Input: part model. Units: mm. Frame: model coordinates. Face numbers are marked on the shaded views. Give positions to 0.01 mm unless a question says otherwise; leave off trailing zeros. Loops run counter-clockwise (first coordinate to the right, second up) from the corner with the lowest first, then second, coordinate; pieces in that order, holes last. Notation, with made-up numbers: (-10.75, -38) - (-6.75, -38) arc R22 ccw to (-6.75, -22) - close; hole circle Ø5 at (64, 57). An arc over 180 degrees is marked (long way). Answer as a JSON object with one key per item and string values.
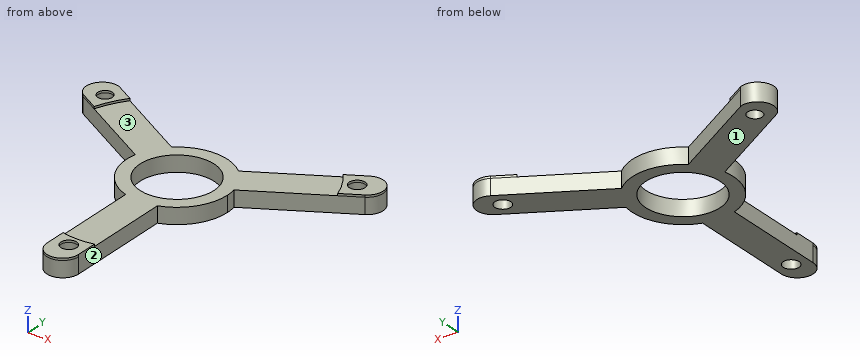
from build123d import *

# Parameters (mm, degrees)
F1_R     = 7.0078592828
F2_DEPTH = 3
F3_R     = 1.3785641614
F3_R_2   = 1.5
F4_DEPTH = 25
F5_R     = 1.3785641614
F5_R_2   = 1.5
F6_DEPTH = 0.4


# Not quite as in the source:
# - a feature names something its author has since deleted; it is built from what else it names


with BuildPart() as f2:
    # F1 (on Top) → F2 (new body)
    with BuildSketch(Plane.XY):
        with BuildLine():
            ThreePointArc((6.3250837122, 7.115890399), (8.2451158332, 4.7603198458), (9.3250837122, 1.9197379763))
            Line((9.3250837122, 1.9197379763), (26.6455917878, 11.9197379763))
            ThreePointArc((26.6455917878, 11.9197379763), (27.7436679992, 16.0178141876), (23.6455917878, 17.115890399))
            Line((23.6455917878, 17.115890399), (6.3250837122, 7.115890399))
        make_face()
        with BuildLine():
            Line((3, -29.0356283753), (3, -9.0356283753))
            ThreePointArc((3, -9.0356283753), (0, -9.5206396916), (-3, -9.0356283753))
            Line((-3, -9.0356283753), (-3, -29.0356283753))
            ThreePointArc((-3, -29.0356283753), (0, -32.0356283753), (3, -29.0356283753))
        make_face()
        with BuildLine():
            ThreePointArc((3, -9.0356283753), (7.7202493228, -5.5713849742), (9.5206396916, 0))
            ThreePointArc((9.5206396916, 0), (9.4716245242, 0.9648362606), (9.3250837122, 1.9197379763))
            ThreePointArc((9.3250837122, 1.9197379763), (8.2451158332, 4.7603198458), (6.3250837122, 7.115890399))
            ThreePointArc((6.3250837122, 7.115890399), (0, 9.5206396916), (-6.3250837122, 7.115890399))
            ThreePointArc((-6.3250837122, 7.115890399), (-8.2451158332, 4.7603198458), (-9.3250837122, 1.9197379763))
            ThreePointArc((-9.3250837122, 1.9197379763), (-8.2451158332, -4.7603198458), (-3, -9.0356283753))
            ThreePointArc((-3, -9.0356283753), (0, -9.5206396916), (3, -9.0356283753))
        make_face()
        Circle(F1_R, mode=Mode.SUBTRACT)
        with BuildLine():
            ThreePointArc((-9.3250837122, 1.9197379763), (-8.2451158332, 4.7603198458), (-6.3250837122, 7.115890399))
            Line((-6.3250837122, 7.115890399), (-23.6455917878, 17.115890399))
            ThreePointArc((-23.6455917878, 17.115890399), (-27.3659550895, 15.7997415376), (-26.6455917878, 11.9197379763))
            Line((-26.6455917878, 11.9197379763), (-9.3250837122, 1.9197379763))
        make_face()
    extrude(amount=F2_DEPTH)

    # F3 (on face) → F4 (cut)
    with BuildSketch(Plane.XY.offset(3)):
        with Locations((-23.8184579752, 13.7452195212)):
            Circle(F3_R)
        with Locations((23.8028700918, 13.7721957361)):
            Circle(F3_R_2)
        with Locations((0, -27.5)):
            Circle(F3_R_2)
    extrude(amount=-F4_DEPTH, mode=Mode.SUBTRACT)

    # F5 (on face) → F6 (join)
    with BuildSketch(Plane.XY.offset(3)):
        with BuildLine():
            ThreePointArc((-22.963211557, 9.7937147588), (-21.7607776153, 12.554595023), (-20.1298891441, 15.0860985312))
            Line((-20.1298891441, 15.0860985312), (-23.6455917878, 17.115890399))
            ThreePointArc((-23.6455917878, 17.115890399), (-27.3659550895, 15.7997415376), (-26.6455917878, 11.9197379763))
            Line((-26.6455917878, 11.9197379763), (-22.963211557, 9.7937147588))
        make_face()
        with Locations((-23.8184579752, 13.7452195212)):
            Circle(F5_R, mode=Mode.SUBTRACT)
        with BuildLine():
            Line((23.6455917878, 17.115890399), (20.1200227065, 15.0804021408))
            ThreePointArc((20.1200227065, 15.0804021408), (21.8423336439, 12.6055758249), (23.0431293377, 9.839855311))
            Line((23.0431293377, 9.839855311), (26.6455917878, 11.9197379763))
            ThreePointArc((26.6455917878, 11.9197379763), (27.7436679992, 16.0178141876), (23.6455917878, 17.115890399))
        make_face()
        with Locations((23.8028700918, 13.7721957361)):
            Circle(F5_R_2, mode=Mode.SUBTRACT)
        with BuildLine():
            ThreePointArc((3, -25.020474568), (-0.0045904533, -25.3057184102), (-3, -24.9363277107))
            Line((-3, -24.9363277107), (-3, -29.0356283753))
            ThreePointArc((-3, -29.0356283753), (0, -32.0356283753), (3, -29.0356283753))
            Line((3, -29.0356283753), (3, -25.020474568))
        make_face()
        with Locations((0, -27.5)):
            Circle(F5_R_2, mode=Mode.SUBTRACT)
    extrude(amount=F6_DEPTH)


solid = f2.part
Item 1: Cut plane B-B (x = -5.5). Return loops of the section in (y, z).
Geometry check:
{"outline": "(-7.77, 0) - (-4.34, 0) - (-4.34, 3) - (-7.77, 3) - close; (4.34, 0) - (7.77, 0) - (7.77, 3) - (4.34, 3) - close"}
Item 2: Cut plane A-A (y = -27.5). Return loops of the section in (x, z).
Geometry check:
{"outline": "(-3, 0) - (-1.5, 0) - (-1.5, 3.4) - (-3, 3.4) - close; (1.5, 0) - (3, 0) - (3, 3.4) - (1.5, 3.4) - close"}
Item 3: Cut plane C-C (z = 1.1). Return loops of the section in (x, y).
Geometry check:
{"outline": "(-26.65, 11.92) - (-9.33, 1.92) arc R9.52 ccw to (-3, -9.04) - (-3, -29.04) arc R3 ccw to (3, -29.04) - (3, -9.04) arc R9.52 ccw to (9.33, 1.92) - (26.65, 11.92) arc R3 ccw to (23.65, 17.12) - (6.33, 7.12) arc R9.52 ccw to (-6.33, 7.12) - (-23.65, 17.12) arc R3.04 ccw to start; hole circle Ø2.76 at (-23.82, 13.75); hole circle Ø14.02 at (0, 0); hole circle Ø3 at (0, -27.5); hole circle Ø3 at (23.8, 13.77)"}
Item 4: Material intervals for line 1 (Y direction, x = 0, z = 0.7); line 2 (X direction, y = 13.5, z = 3.25); line 3 (X direction, y = 13, z = 2.7), sorted ascending. Write a range as [from, to].
Geometry check:
{"line 1": "y = [-32.04, -29], [-26, -7.01], [7.01, 9.52]", "line 2": "x = [-27.67, -25.18], [-22.46, -21.22], [21.3, 22.33], [25.28, 27.97]", "line 3": "x = [-27.49, -24.98], [-22.66, -16.52], [16.52, 22.52], [25.09, 27.73]"}
Item 5: Cut plane D-D (y = 13). Return loops of the section in (x, z), then the cut area to 3 significant figures.
Geometry check:
{"outline": "(-27.49, 0) - (-24.98, 0) - (-24.98, 3.4) - (-27.49, 3.4) - close; (-22.66, 0) - (-16.52, 0) - (-16.52, 3) - (-21.51, 3) - (-21.51, 3.4) - (-22.66, 3.4) - close; (16.52, 0) - (22.52, 0) - (22.52, 3.4) - (21.61, 3.4) - (21.61, 3) - (16.52, 3) - close; (25.09, 0) - (27.73, 0) - (27.73, 3.4) - (25.09, 3.4) - close", "area": "54.8 mm2"}
Item 6: Mould query, pull axis X, two halves, no side actions, for the marked faces 1, 2 and 3. Classes: released by +X, released by -X, zero draft, split by the parting line, or undercut.
Geometry check:
{"face 1": "zero draft", "face 2": "released by +X", "face 3": "undercut"}
Item 7: Contact query for flat-ended pins moving along their axis: P1, Ø1, axis at y = -6, z = 2, coming from the -X side; P2, Ø1.5, axis at x = 9, z = 2, coming from the -Y side; P3, Ø1.5, axis at x = 17, z = 0.5, coming from the -Y side. Output: stop coordinate, or through.
Geometry check:
{"P1": "stops at x = -7.77", "P2": "stops at y = -4.75", "P3": "stops at y = 5.92"}
